```python
from build123d import *

# Parameters (mm, degrees)
PAD_DEPTH    = 40
SKETCH001_R  = 5
POCKET_DEPTH = 50.001


with BuildPart() as part:
    # Sketch → Pad (new body)
    with BuildSketch(Plane.XZ):
        with BuildLine():
            Line((0, 0), (110, 0))
            Line((110, 0), (110, 30))
            ThreePointArc((110, 30), (104.142136, 44.142136), (90, 50))
            Line((50, 50), (90, 50))
            Line((0, 21.132487), (50, 50))
            Line((0, 0), (0, 21.132487))
        make_face()
    extrude(amount=PAD_DEPTH)

    # Sketch001 (on Face4 of Pad) → Pocket (cut, through all)
    with BuildSketch(Plane(origin=(0, 0, 50), x_dir=(-1, 0, 0), z_dir=(0, 0, 1))):
        with Locations((-70, 20)):
            Circle(SKETCH001_R)
    extrude(amount=-POCKET_DEPTH, mode=Mode.SUBTRACT)


solid = part.part
```
Work out the finished part from the listing and answer in its coordinate system (mm). Coordinates: 2 decimals unless noted, no trailing zeros. Loops run counter-clockwise (first coordinate to the right, second up) from the corner with the lowest first, then second, coordinate; pieces in that order, holes last. Notation, with made-up numbers: (-0.75, 65.25) - (46.25, 65.25) arc R36 cw to (46.25, 103.25) - close; hole circle Ø9 at (36, -38.75). An arc over 180 degrees is marked (long way). Use a Markdown table: item, result.
Item 1: Find section B-B, the plane y = -20. Determine the outline of the cut face in (x, z), and give its area (3 significant figures).
Evaluation:
| item | result |
|---|---|
| outline | (0, 0) - (65, 0) - (65, 50) - (50, 50) - (0, 21.13) - close; (75, 0) - (110, 0) - (110, 30) arc R20 ccw to (90, 50) - (75, 50) - close |
| area | 4,190 mm2 |
Item 2: Find section D-D, the plane z = 33.5. Determine the outline of the cut face in (x, y).
Evaluation:
| item | result |
|---|---|
| outline | (21.42, -40) - (109.69, -40) - (109.69, 0) - (21.42, 0) - close; hole circle Ø10 at (70, -20) |
Item 3: Find section A-A, the plane x = 70. Determine the outline of the cut face in (y, z).
Evaluation:
| item | result |
|---|---|
| outline | (-40, 0) - (-25, 0) - (-25, 50) - (-40, 50) - close; (-15, 0) - (0, 0) - (0, 50) - (-15, 50) - close |
Item 4: Consider probe 1 along Y at (x, z) = (70, 15); probe 2 along X at (y, z) = (-20, 39.5); probe 3 along X at (y, z) = (-20, 31). Determine where each line is inside the solid, lowest interval first. Write a range as from..to.
Evaluation:
| item | result |
|---|---|
| probe 1 | y = -40..-25, -15..0 |
| probe 2 | x = 31.81..65, 75..107.6 |
| probe 3 | x = 17.09..65, 75..109.97 |
Item 5: Given pin 1 Ø13 at (x, y) = (70, -20) entering from +Z; pin 2 Ø6 at (y, z) = (-24.5, 30) entering from -X, each flat-ended and moving along its own axis, determine where each tip first touches the part or whether it passes through.
Evaluation:
| item | result |
|---|---|
| pin 1 | stops at z = 50 |
| pin 2 | stops at x = 10.16 |
Item 6: The mould has two halves that part along Y. Classify faces 1 (the cylindrical face through (65.381, -18.085, 25.35)), 2 (the flat face through (54, 0, 25)), 3 (the flat face through (54, -20, 0)): +Y half, -Y half, draft (parallel to the pull), parting line (faces both ways), or undercut.
Evaluation:
| item | result |
|---|---|
| face 1 | undercut |
| face 2 | +Y half |
| face 3 | draft |
Item 7: Find section C-C, the plane y = -29. Determine the outline of the cut face in (x, z), and give its area (3 significant figures).
Evaluation:
| item | result |
|---|---|
| outline | (0, 0) - (110, 0) - (110, 30) arc R20 ccw to (90, 50) - (50, 50) - (0, 21.13) - close |
| area | 4,690 mm2 |
